Verification items for the finished model (mm, model axes). Give positions to 0.01 mm unless a question says otherwise; leave off trailing zeros. Write each loop counter-clockwise with the first axis right and the second up, starting at its lowest first coordinate (ties: lowest second). Pieces come first, ordered by that corner, then holes.
from build123d import *

# Parameters (mm, degrees)
F0_W          = 88.9
F0_H          = 19.05
F1_DEPTH      = 406.4
F3_DEPTH      = 4.7625
F3_DEPTH_BACK = 4.7625


# Not quite as in the source:
# - a pattern or mirror of a feature is missing from the dataset's text; its kind, count and spacing are read off the source's solid


with BuildPart() as f1:
    # F0 (on Right) → F1 (new body)
    with BuildSketch(Plane.YZ):
        Rectangle(F0_W, F0_H)
    extrude(amount=F1_DEPTH)

    # F2 (on Top) → F3 (cut, two sides)
    with BuildSketch(Plane.XY) as f3_sk:
        with BuildLine():
            Line((0, 31.75), (0, -31.75))
            ThreePointArc((0, -31.75), (12.7, 0), (0, 31.75))
        make_face()
    f3 = extrude(amount=F3_DEPTH, mode=Mode.SUBTRACT) + extrude(f3_sk.sketch, amount=-F3_DEPTH_BACK, mode=Mode.SUBTRACT)

    # F3_copies: F3 across plane
    add(f3.mirror(Plane(origin=(203.2, 0, 0), x_dir=(0, 0, 1), z_dir=(1, 0, 0))), mode=Mode.SUBTRACT)


solid = f1.part
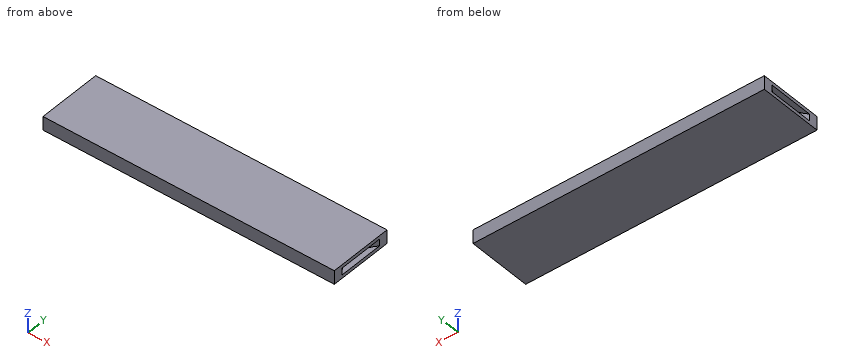
Item 1: Depth check by flat-ended pin: pin 1 (1.5 mm diameter, centred on y = 7.5, z = 0.5, fed in from -X). Enter the tip coordinate at first touch or a pass-through.
Answer key:
pin 1: stops at x = 11.95
Item 2: Sectioned sample at B-B on y = -12.5. Record the cut outline in (x, z) (1 decimal), then the cut area to 3 significant figures.
Answer key:
outline: (0, -9.5) - (406.4, -9.5) - (406.4, -4.8) - (395.4, -4.8) - (395.4, 4.8) - (406.4, 4.8) - (406.4, 9.5) - (0, 9.5) - (0, 4.8) - (11, 4.8) - (11, -4.8) - (0, -4.8) - close
area: 7,530 mm2
Item 3: Sectioned sample at C-C on y = 8.5. Record the cut outline in (x, z) (1 decimal).
Answer key:
outline: (0, -9.5) - (406.4, -9.5) - (406.4, -4.8) - (394.5, -4.8) - (394.5, 4.8) - (406.4, 4.8) - (406.4, 9.5) - (0, 9.5) - (0, 4.8) - (11.9, 4.8) - (11.9, -4.8) - (0, -4.8) - close
Item 4: Scan lines: line 1 along X through (y, z) = (-23, 1); line 2 along X through (y, z) = (-6, 3.5). Record each from-to range of solid material in increasing order.
Answer key:
line 1: x = 6.54 to 399.86
line 2: x = 12.31 to 394.09
